from build123d import *

# Parameters (mm, degrees)
SKETCH002_W  = 100
SKETCH002_H  = 80
SKETCH002_R  = 1.75
PAD004_DEPTH = 3.4
SKETCH_W     = 80
SKETCH_H     = 51
POCKET_DEPTH = 5
CHAMFER_SIZE = 1.5
FILLET_R     = 1.5


with BuildPart() as part:
    # Sketch002 → Pad004 (new body)
    with BuildSketch(Plane.XY.offset(49.5)):
        with Locations((-14.266246, -4.330319)):
            Rectangle(SKETCH002_W, SKETCH002_H)
        with Locations((-59.499317, 30.08403)):
            Circle(SKETCH002_R, mode=Mode.SUBTRACT)
        with Locations((-59.584126, -34.915915)):
            Circle(SKETCH002_R, mode=Mode.SUBTRACT)
        with Locations((28.500684, 29.937426)):
            Circle(SKETCH002_R, mode=Mode.SUBTRACT)
        with Locations((28.415874, -35.062521)):
            Circle(SKETCH002_R, mode=Mode.SUBTRACT)
    extrude(amount=PAD004_DEPTH)

    # Sketch (on Face10 of Pad004) → Pocket (cut)
    with BuildSketch(Plane.XY.offset(52.9)):
        with Locations((-14.266246, -4.830319)):
            Rectangle(SKETCH_W, SKETCH_H)
    extrude(amount=-POCKET_DEPTH, mode=Mode.SUBTRACT)

    # Chamfer
    chamfer_edges = [part.edges().sort_by_distance(p)[0] for p in [
        (-61.334126, -34.915915, 52.9),
        (-61.249317, 30.08403, 52.9),
        (26.750684, 29.937426, 52.9),
        (26.665874, -35.062521, 52.9),
    ]]
    chamfer(chamfer_edges, length=CHAMFER_SIZE)

    # Fillet
    fillet_edges = [part.edges().sort_by_distance(p)[0] for p in [
        (-64.266246, -4.330319, 52.9),
        (-14.266246, -44.330319, 52.9),
        (35.733754, -4.330319, 52.9),
        (-14.266246, 35.669681, 52.9),
    ]]
    fillet(fillet_edges, radius=FILLET_R)


solid = part.part
Read the model definition and answer for the solid it produces. Units are mm, in the model's axes. A direction names the side the tool comes from. Give positions to 0.01 mm unless a question says otherwise; leave off trailing zeros. Loops run counter-clockwise (first coordinate to the right, second up) from the corner with the lowest first, then second, coordinate; pieces in that order, holes last. Notation, with made-up numbers: (-4, -22) -> (36, -22) arc R15 ccw to (36, -9) -> close; hole circle Ø11 at (74.5, 44.25). An arc over 180 degrees is marked (long way). Use a Markdown table: item, result.
Q1. Determine the mould class of faces 3 (the face through (-15, -30.33, 51)), 4 (the face through (-15, 23, 49.5)) for opening direction Y: pulls with the +Y half, pulls with the -Y half, needs draft (parallel to the pull), parting line crosses it, or undercut.
Solved:
| item | result |
|---|---|
| face 3 | undercut |
| face 4 | needs draft |
Q2. Find the intervals of material crossed by line 1 along X through (y, z) = (-35, 51.1); line 2 along X through (y, z) = (-15, 51.65); line 3 along X through (y, z) = (-14, 49.95), in increasing order.
Solved:
| item | result |
|---|---|
| line 1 | x = -64.27 to -61.33, -57.84 to 26.67, 30.16 to 35.73 |
| line 2 | x = -64.25 to -54.27, 25.73 to 35.71 |
| line 3 | x = -64.27 to -54.27, 25.73 to 35.73 |
Q3. A tool of negligible diameter and unlimited length cuts with its end or side. For faces 1 (the face through (-15, 22, 52.9)), 2 (the face through (-54.266, -5, 51)), from which of +Z, -Z, +X, -X, +Y, -Y can it reach the whole face along a straight path? Write none if from no direction.
Solved:
| item | result |
|---|---|
| face 1 | +Z, +X, -X, +Y, -Y |
| face 2 | +Z, -Z |
Q4. This flat-tipped pin is pushed along its axis until it touches: pin 1 (5.5 mm diameter, centred on x = -59.58, y = -34.92, fed in from -Z). Where does it stop, or does it pass through?
Solved:
| item | result |
|---|---|
| pin 1 | stops at z = 49.5 |
Q5. Section C-C, the plane z = 50.3 is taken. Determine the outline of the cut face in (x, y), then the cut area to 3 significant figures.
Solved:
| item | result |
|---|---|
| outline | (-64.27, -44.33) -> (35.73, -44.33) -> (35.73, 35.67) -> (-64.27, 35.67) -> close; hole circle Ø3.5 at (-59.58, -34.92); hole circle Ø3.5 at (-59.5, 30.08); hole (-54.27, -30.33) -> (25.73, -30.33) -> (25.73, 20.67) -> (-54.27, 20.67) -> close; hole circle Ø3.5 at (28.42, -35.06); hole circle Ø3.5 at (28.5, 29.94) |
| area | 3,880 mm^2 |
Q6. Section B-B, the plane y = 9 is taken. Determine the outline of the cut face in (x, z).
Solved:
| item | result |
|---|---|
| outline | (-64.27, 49.5) -> (-54.27, 49.5) -> (-54.27, 52.9) -> (-62.77, 52.9) arc R1.5 ccw to (-64.27, 51.4) -> close; (25.73, 49.5) -> (35.73, 49.5) -> (35.73, 51.4) arc R1.5 ccw to (34.23, 52.9) -> (25.73, 52.9) -> close |
Q7. Section A-A, the plane x = -10 is taken. Determine the outline of the cut face in (y, z), then the cut area to 3 significant figures.
Solved:
| item | result |
|---|---|
| outline | (-44.33, 49.5) -> (-30.33, 49.5) -> (-30.33, 52.9) -> (-42.83, 52.9) arc R1.5 ccw to (-44.33, 51.4) -> close; (20.67, 49.5) -> (35.67, 49.5) -> (35.67, 51.4) arc R1.5 ccw to (34.17, 52.9) -> (20.67, 52.9) -> close |
| area | 97.6 mm^2 |
